```python
from build123d import *

# Parameters (mm, degrees)
PAD_DEPTH       = 36
SKETCH001_W     = 41.77589
SKETCH001_H     = 47.890068
POCKET_DEPTH    = 10.5
SKETCH002_R     = 2.75
POCKET001_DEPTH = 36.001
FILLET_R        = 4
FILLET001_R     = 0.5
SKETCH003_R     = 2.85
HOLE_DEPTH      = 16.001
FILLET002_R     = 6
CHAMFER_SIZE    = 2
POCKET002_DEPTH = 3


with BuildPart() as part:
    # Sketch → Pad (new body)
    with BuildSketch(Plane.XZ):
        with BuildLine():
            Line((-20, 0), (20, 0))
            Line((20, 10), (20, 0))
            Line((10, 10), (20, 10))
            Line((10, 30), (10, 10))
            ThreePointArc((10, 30), (0, 40), (-10, 30))
            Line((-10, 10), (-10, 30))
            Line((-20, 10), (-10, 10))
            Line((-20, 0), (-20, 10))
        make_face()
    extrude(amount=PAD_DEPTH)

    # Sketch001 (on DatumPlane) → Pocket (cut, symmetric)
    with BuildSketch(Plane(origin=(0, -18, 0), x_dir=(1, 0, 0), z_dir=(0, 1, 0))):
        with Locations((0.131337, -38.945034)):
            Rectangle(SKETCH001_W, SKETCH001_H)
    extrude(amount=POCKET_DEPTH, both=True, mode=Mode.SUBTRACT)

    # Sketch002 (on Face4 of Pocket) → Pocket001 (cut, through all)
    with BuildSketch(Plane(origin=(0, 0, 0), x_dir=(1, 0, 0), z_dir=(0, 1, 0))):
        with Locations((0, -30)):
            Circle(SKETCH002_R)
    extrude(amount=-POCKET001_DEPTH, mode=Mode.SUBTRACT)

    # Fillet
    fillet_edges = [part.edges().sort_by_distance(p)[0] for p in [
        (10, -18, 15),
        (-10, -18, 15),
    ]]
    fillet(fillet_edges, radius=FILLET_R)

    # Fillet001
    fillet001_edges = [part.edges().sort_by_distance(p)[0] for p in [
        (10, -18, 10),
        (-10, -18, 10),
    ]]
    fillet(fillet001_edges, radius=FILLET001_R)

    # Sketch003 (on DatumPlane) → Hole (cut, through all)
    with BuildSketch(Plane(origin=(0, 0, 16), x_dir=(1, 0, 0), z_dir=(0, 0, -1))):
        with Locations((15, 18)):
            Circle(SKETCH003_R)
        with Locations((-15, 18)):
            Circle(SKETCH003_R)
    extrude(amount=HOLE_DEPTH, mode=Mode.SUBTRACT)

    # Fillet002
    fillet002_edges = [part.edges().sort_by_distance(p)[0] for p in [
        (20, 0, 5),
        (-20, 0, 5),
        (-20, -36, 5),
        (20, -36, 5),
    ]]
    fillet(fillet002_edges, radius=FILLET002_R)

    # Chamfer
    chamfer_edges = [part.edges().sort_by_distance(p)[0] for p in [
        (-2.75, 0, 30),
    ]]
    chamfer(chamfer_edges, length=CHAMFER_SIZE)

    # Sketch004 (on Face15 of Chamfer) → Pocket002 (cut)
    with BuildSketch(Plane.XZ.offset(36)):
        Polygon((-0.093793, 34.5), (-3.944011, 32.168773), (-3.850218, 27.668773), (0.093793, 25.5), (3.944011, 27.831227), (3.850218, 32.331227), align=None)
    extrude(amount=-POCKET002_DEPTH, mode=Mode.SUBTRACT)


solid = part.part
```
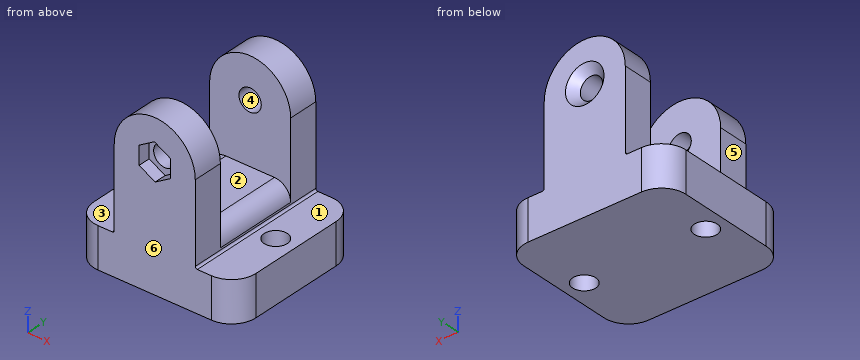
Can you work these out from the model? Positions are in its coordinate system, mm. Face numbers are marked on the shaded views. A direction names the side the tool comes from. Coordinates: 2 decimals unless noted, no trailing zeros. Loops run counter-clockwise (first coordinate to the right, second up) from the corner with the lowest first, then second, coordinate; pieces in that order, holes last. Notation, with made-up numbers: (53, -38) - (81, -38) arc R28 ccw to (81, -19) - close; hole circle Ø7 at (-15, 66.25). An arc over 180 degrees is marked (long way). Use a Markdown table: item, result.
Item 1: I want a section at B-B on x = 15. Please give me the cut outline in (y, z).
Numbers:
| item | result |
|---|---|
| outline | (-35.92, 0) - (-20.85, 0) - (-20.85, 10) - (-35.92, 10) - close; (-15.15, 0) - (-0.08, 0) - (-0.08, 10) - (-15.15, 10) - close |
Item 2: I want a section at A-A on y = -18. Please give me the cut outline in (x, z).
Numbers:
| item | result |
|---|---|
| outline | (-20, 0) - (-17.85, 0) - (-17.85, 10) - (-20, 10) - close; (-12.15, 0) - (12.15, 0) - (12.15, 10) - (10.5, 10) arc R0.5 cw to (10, 10.5) - (10, 11) arc R4 ccw to (6, 15) - (-6, 15) arc R4 ccw to (-10, 11) - (-10, 10.5) arc R0.5 cw to (-10.5, 10) - (-12.15, 10) - close; (17.85, 0) - (20, 0) - (20, 10) - (17.85, 10) - close |
Item 3: I want a section at C-C on z = 3. Please give me the cut outline in (x, y).
Numbers:
| item | result |
|---|---|
| outline | (-20, -30) arc R6 ccw to (-14, -36) - (14, -36) arc R6 ccw to (20, -30) - (20, -6) arc R6 ccw to (14, 0) - (-14, 0) arc R6 ccw to (-20, -6) - close; hole circle Ø5.7 at (-15, -18); hole circle Ø5.7 at (15, -18) |
Item 4: I want a section at D-D on y = -5. Please give me the cut outline in (x, z), and give its area (3 significant figures).
Numbers:
| item | result |
|---|---|
| outline | (-19.92, 0) - (19.92, 0) - (19.92, 10) - (10.5, 10) arc R0.5 cw to (10, 10.5) - (10, 30) arc R10 ccw to (-10, 30) - (-10, 10.5) arc R0.5 cw to (-10.5, 10) - (-19.92, 10) - close; hole circle Ø5.5 at (0, 30) |
| area | 932 mm2 |
Item 5: If I drill on probe 1 along Z at (x, y) = (0, -32.1); probe 2 along Y at (x, z) = (6, 20); probe 3 along Z at (x, y) = (-10.5, -15.5), over which ranges is the centre line in solid material (lowest first)? Write a range as from..to.
Numbers:
| item | result |
|---|---|
| probe 1 | z = 0..27.25, 32.75..40 |
| probe 2 | y = -36..-28.5, -7.5..0 |
| probe 3 | z = 0..10 |
Item 6: For the marked faces 1, 2 and 3, which set-ups out of +Z, -Z, +X, -X, +Y, -Y let a thin tool reach every point of the face, with its end or its side?
Numbers:
| item | result |
|---|---|
| face 1 | +Z, +X, +Y, -Y |
| face 2 | +Z, +X, -X |
| face 3 | +Z, -X, +Y, -Y |
Item 7: Will these pins go through, and if not, where does the flat tip stop? pin 1 (7.5 mm diameter, centred on x = -14.5, y = -18.5, fed in from +Z); pin 2 (10 mm diameter, centred on y = -15, z = 19.5, fed in from -X); pin 3 (6 mm diameter, centred on y = -4.5, z = 22.5, fed in from +X); pin 4 (5 mm diameter, centred on x = 15, y = -18, fed in from -Z).
Numbers:
| item | result |
|---|---|
| pin 1 | stops at z = 10 |
| pin 2 | stops at x = -7.94 |
| pin 3 | stops at x = 10 |
| pin 4 | passes through |
Item 8: We'd pull the mould along X, two halves only. Please class the marked faces 4, 5 and 6: released by +X, released by -X, zero draft, split by the parting line, or undercut.
Numbers:
| item | result |
|---|---|
| face 4 | undercut |
| face 5 | released by -X |
| face 6 | zero draft |
